Design review of the part shown in the three views and the two pictorial views. Dimensions are in mm from the part's minimum x, y and z. Round coordinates to 2 decimals unless told otherwise and drop trailing zeros. Loops run counter-clockwise (first coordinate to the right, second up) from the corner with the lowest first, then second, coordinate; pieces in that order, holes last. Notation, with made-up numbers: M 83,65 L 91,65 A15 cw 91,81 Z; hole C -19.5,6.5 d11. An arc over 180 degrees is marked long. One line per question, with ' | ' between items.
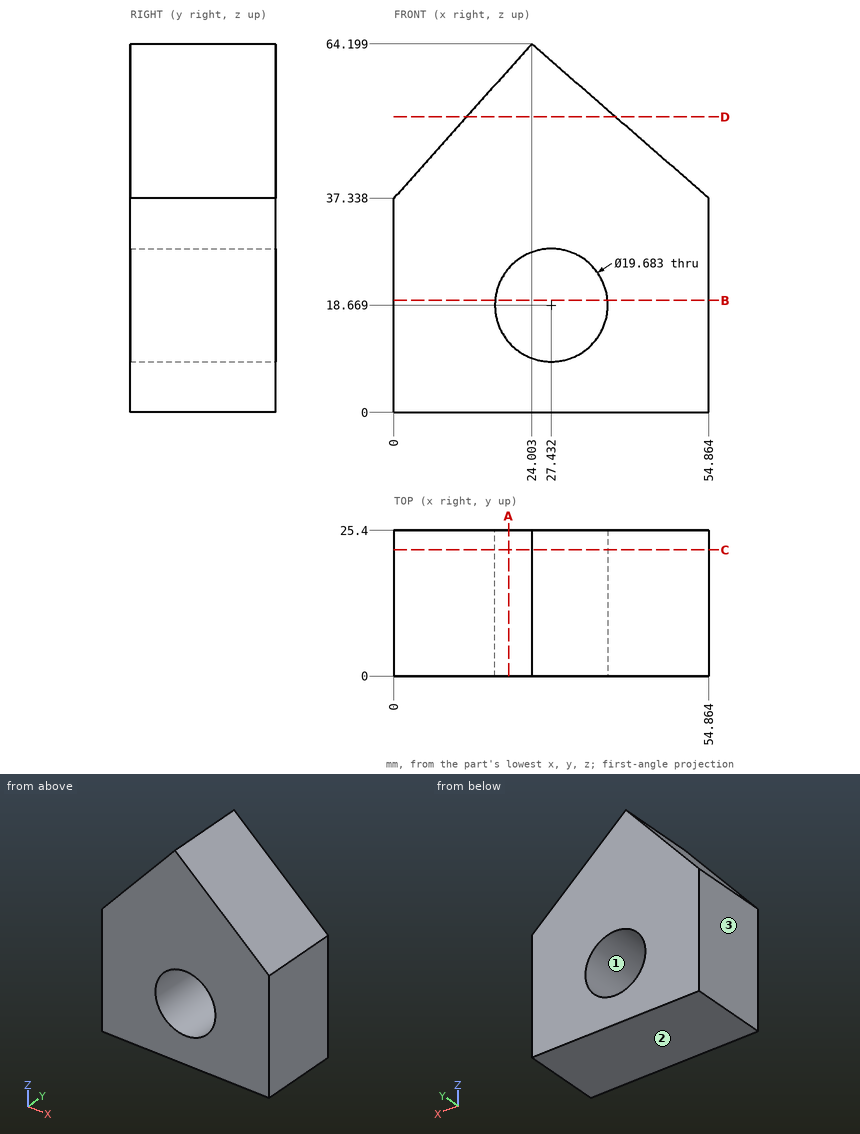
1) Add section C-C on y = 22. State the section outline as (x, z) points (1 decimal).
Output values:
outline: M 0,0 L 54.9,0 L 54.9,37.3 L 24,64.2 L 0,37.3 Z; hole C 27.4,18.7 d19.7
2) Add section A-A on x = 20. State the section outline as (y, z) points, then the cut area to 3 significant figures.
Output values:
outline: M 0,0 L 25.4,0 L 25.4,12.22 L 0,12.22 Z; M 0,25.12 L 25.4,25.12 L 25.4,59.72 L 0,59.72 Z | area: 1,190 mm²
3) For line 1 (X direction, y = 17.25, z = 26.5) (1 decimal); line 2 (Z direction, x = 36, y = 18.75) (1 decimal); line 3 (Z direction, x = 24, y = 18.25) (1 decimal), list the stretches that pass through material, from the lowest coordinate up.
Output values:
line 1: x = 0 to 21.5, 33.4 to 54.9 | line 2: z = 0 to 13.8, 23.5 to 53.8 | line 3: z = 0 to 9.4, 27.9 to 64.2
4) Insertion check: P1, Ø1.5, axis at y = 19, z = 57, coming from the -X side; P2, Ø10, axis at x = 21, y = 5, coming from the +Z side. Each pin has a flat end and moves straight along its axis. Give the tip position at first contact, or say it passes through.
Output values:
P1: stops at x = 16.9 | P2: stops at z = 64.2
5) Add section D-D on z = 51.5. State the section outline as (x, y) points (1 decimal).
Output values:
outline: M 12.7,0 L 38.6,0 L 38.6,25.4 L 12.7,25.4 Z
6) Add section B-B on z = 19.5. State the section outline as (x, y) points (1 decimal).
Output values:
outline: M 0,0 L 17.6,0 L 17.6,25.4 L 0,25.4 Z; M 37.2,0 L 54.9,0 L 54.9,25.4 L 37.2,25.4 Z
7) Mouldability with a two-part tool opening along X and no side actions: class the marked faces 1, 2 and 3 as +X half, -X half, draft (parallel to the pull), parting line (faces both ways), or undercut.
Output values:
face 1: undercut | face 2: draft | face 3: -X half
